Can you work these out from the model? Positions are in its coordinate system, mm. Give positions to 0.01 mm unless a question says otherwise; leave off trailing zeros. Write each loop counter-clockwise with the first axis right and the second up, starting at its lowest first coordinate (ties: lowest second). Pieces come first, ordered by that corner, then holes.
1. If I drill on probe 1 along Y at (x, z) = (0, -6.3); probe 2 along X at (y, z) = (60.5, 0.75); probe 3 along Z at (x, y) = (1, 393.5), over which ranges is the centre line in solid material (lowest first)?
2. Suppose I cut it at A-A (z = 0). Please give me the cut outline in (x, y), and give its area (3 significant figures).
3. I'm going to push flat-ended pins straight in: pin 1 (3 mm diameter, centred on y = 457.5, z = -2.5, fed in from -X); pin 2 (1 mm diameter, centred on x = -3, y = 161.5, fed in from +Z); pin 3 (8 mm diameter, centred on y = 246, z = 4.5, fed in from -X). Where does each tip first touch, or does it pass through?
4. Suppose I cut it at B-B (y = 107). Please give me the cut outline in (x, z).
5. Thinking about a two-plate mould opening in Z: for faces 1 (the cylindrical face through (1.802, 283.92, -5.723)), 2 (the cylindrical face through (-6.834, 276.08, -1.517)), 3 (the flat face through (2, 0, 6)), which applies, pulls with the +Z half, pulls with the -Z half, needs draft (parallel to the pull), parting line crosses it, or undercut?
```python
from build123d import *

# Parameters (mm, degrees)
SKETCH_1_R               = 7
EXTRUDE_1_DEPTH          = 560
CUT_EXTRUDE_1_DEPTH      = 561.087493165
CUT_EXTRUDE_1_DEPTH_BACK = 561.087493165
SKETCH_2_R               = 6
HOLE_WIZARD_M2_5_1_D     = 2.9


with BuildPart() as part:
    # 스케치1 → 보스-돌출1 (new body)
    with BuildSketch(Plane(origin=(0, 0, 0), x_dir=(1, 0, 0), z_dir=(0, 1, 0))):
        with Locations(Location((0, 0, 0), (0, 0, 270))):
            Circle(SKETCH_1_R)
    extrude(amount=EXTRUDE_1_DEPTH)

    # 스케치2 → 컷-돌출1 (cut, two sides: drawn at the far end of the back side and taken through both)
    with BuildSketch(Plane.XZ.offset(-CUT_EXTRUDE_1_DEPTH_BACK)):
        with Locations(Location((0, 0, 0), (0, 0, 270))):
            Circle(SKETCH_2_R)
    extrude(amount=CUT_EXTRUDE_1_DEPTH + CUT_EXTRUDE_1_DEPTH_BACK, mode=Mode.SUBTRACT)

    # M2.5 여유 구멍1 (through all)
    with Locations(Plane.XY.offset(7)):
        with Locations((0, 18), (0, 542)):
            Hole(HOLE_WIZARD_M2_5_1_D / 2)


solid = part.part
```
Checks:
1. probe 1: y = 0 to 16.55, 19.45 to 540.55, 543.45 to 560
1. probe 2: x = -6.96 to -5.95, 5.95 to 6.96
1. probe 3: z = -6.93 to -5.92, 5.92 to 6.93
2. outline: (-7, 0) - (-6, 0) - (-6, 560) - (-7, 560) - close; (6, 0) - (7, 0) - (7, 560) - (6, 560) - close
2. area: 1,120 mm2
3. pin 1: stops at x = -6.93
3. pin 2: stops at z = 6.54
3. pin 3: stops at x = -6.98
4. outline: circle Ø14 at (0, 0); hole circle Ø12 at (0, 0)
5. face 1: undercut
5. face 2: parting line crosses it
5. face 3: needs draft
